Can you work these out from the model? Positions are in its coordinate system, mm. A direction names the side the tool comes from. Give positions to 0.01 mm unless a question says otherwise; leave off trailing zeros. Loops run counter-clockwise (first coordinate to the right, second up) from the corner with the lowest first, then second, coordinate; pieces in that order, holes last. Notation, with made-up numbers: (-39.75, 33.25) - (-33.75, 33.25) arc R23 ccw to (-33.75, 72.25) - close; hole circle Ø3 at (77, 37.25). An arc over 180 degrees is marked (long way). Answer as a JSON object with one key per item and string values.
```python
from build123d import *

# Parameters (mm, degrees)
SKETCH1_R                = 25
SKETCH1_R_2              = 16
BOSS_EXTRUDE1_DEPTH      = 45
BOSS_EXTRUDE2_DEPTH      = 10
BOSS_EXTRUDE3_DEPTH      = 35
FILLET1_R                = 12
FILLET2_R                = 12
FILLET3_R                = 6
FILLET4_R                = 12
FILLET5_R                = 3
FILLET6_R                = 6
BOSS_EXTRUDE4_DEPTH      = 48
BOSS_EXTRUDE4_DEPTH_BACK = 48
SKETCH2_R                = 19
SKETCH2_R_2              = 10
BOSS_EXTRUDE5_DEPTH      = 45
BOSS_EXTRUDE5_DEPTH_BACK = 45
SKETCH3_W                = 70
SKETCH3_H                = 86.046908332
CUT_EXTRUDE1_DEPTH       = 138.818721515
FILLET7_R                = 6
SKETCH4_R                = 5
CUT_EXTRUDE2_DEPTH       = 132.658649545
SKETCH6_R                = 19
SKETCH6_R_2              = 10
BOSS_EXTRUDE7_DEPTH      = 16
SKETCH7_R                = 19
SKETCH7_R_2              = 10
BOSS_EXTRUDE8_DEPTH      = 16


with BuildPart() as part:
    # Sketch1 → Boss-Extrude1 (new body)
    with BuildSketch(Plane(origin=(0, 0, 0), x_dir=(1, 0, 0), z_dir=(0, 1, 0))):
        with Locations(Location((0, 0, 0), (0, 0, 90))):
            Circle(SKETCH1_R)
        with Locations(Location((0, 0, 0), (0, 0, 90))):
            Circle(SKETCH1_R_2, mode=Mode.SUBTRACT)
    extrude(amount=BOSS_EXTRUDE1_DEPTH)

    # Sketch1<3> → Boss-Extrude2 (add)
    with BuildSketch(Plane(origin=(0, 0, 0), x_dir=(1, 0, 0), z_dir=(0, 1, 0))):
        with BuildLine():
            Line((-45, 50), (-69, 50))
            Line((-69, 50), (-69, 12))
            Line((-69, 12), (-45, 12))
            Line((-45, 12), (-45, -28))
            Line((-45, -28), (45, -28))
            Line((45, -28), (45, 12))
            Line((45, 12), (69, 12))
            Line((69, 12), (69, 50))
            Line((69, 50), (45, 50))
            Line((45, 50), (45, 25))
            Line((45, 25), (25, 25))
            Line((25, 25), (25, 0))
            ThreePointArc((25, 0), (0, -25), (-25, 0))
            Line((-25, 0), (-25, 25))
            Line((-25, 25), (-45, 25))
            Line((-45, 25), (-45, 50))
        make_face()
    extrude(amount=BOSS_EXTRUDE2_DEPTH)

    # Sketch1<4> → Boss-Extrude3 (add)
    with BuildSketch(Plane(origin=(0, 0, 0), x_dir=(1, 0, 0), z_dir=(0, 1, 0))):
        with BuildLine():
            Line((-35, 35), (-35, 60))
            Line((-35, 60), (-75, 60))
            Line((-75, 60), (-75, 50))
            Line((-75, 50), (-69, 50))
            Line((-69, 50), (-45, 50))
            Line((-45, 50), (-45, 25))
            Line((-45, 25), (-25, 25))
            Line((-25, 25), (-25, 0))
            ThreePointArc((-25, 0), (0, 25), (25, 0))
            Line((25, 0), (25, 25))
            Line((25, 25), (45, 25))
            Line((45, 25), (45, 50))
            Line((45, 50), (69, 50))
            Line((69, 50), (75, 50))
            Line((75, 50), (75, 60))
            Line((75, 60), (35, 60))
            Line((35, 60), (35, 35))
            Line((35, 35), (-35, 35))
        make_face()
    extrude(amount=BOSS_EXTRUDE3_DEPTH)

    # Fillet1
    fillet1_edges = [part.edges().sort_by_distance(p)[0] for p in [
        (45, 22.5, -25),
        (-45, 22.5, -25),
    ]]
    fillet(fillet1_edges, radius=FILLET1_R)

    # Fillet2
    fillet2_edges = [part.edges().sort_by_distance(p)[0] for p in [
        (-45, 5, -12),
        (45, 5, -12),
    ]]
    fillet(fillet2_edges, radius=FILLET2_R)

    # Fillet3
    fillet3_edges = [part.edges().sort_by_distance(p)[0] for p in [
        (69, 5, -50),
        (-69, 5, -50),
    ]]
    fillet(fillet3_edges, radius=FILLET3_R - 0.0001)  # a hair under: the kernel refuses the full size

    # Fillet4
    fillet4_edges = [part.edges().sort_by_distance(p)[0] for p in [
        (69, 5, -12),
        (-69, 5, -12),
    ]]
    fillet(fillet4_edges, radius=FILLET4_R - 0.0001)  # a hair under: the kernel refuses the full size

    # Fillet5
    fillet5_edges = [part.edges().sort_by_distance(p)[0] for p in [
        (25, 22.5, -25),
        (35, 17.5, -35),
        (-35, 17.5, -35),
        (-25, 22.5, -25),
    ]]
    fillet(fillet5_edges, radius=FILLET5_R)

    # Fillet6
    fillet6_edges = [part.edges().sort_by_distance(p)[0] for p in [
        (45, 22.5, -50),
        (-45, 22.5, -50),
    ]]
    fillet(fillet6_edges, radius=FILLET6_R)



with BuildPart() as body_2:
    # Sketch2 → Boss-Extrude4 (new, two sides: drawn at the far end of the back side and taken through both)
    with BuildSketch(Plane(origin=(0, 0, 0), x_dir=(0, 0, -1), z_dir=(1, 0, 0)).offset(-BOSS_EXTRUDE4_DEPTH_BACK)):
        with Locations((0, -56)):
            Circle(SKETCH2_R)
        with Locations((0, -56)):
            Circle(SKETCH2_R_2, mode=Mode.SUBTRACT)
    extrude(amount=BOSS_EXTRUDE4_DEPTH + BOSS_EXTRUDE4_DEPTH_BACK)


with BuildPart() as part_1:
    add(part.part)

    add(body_2.part)  # Boss-Extrude5 merges body 2
    # Sketch2<4> → Boss-Extrude5 (add, two sides: drawn at the far end of the back side and taken through both)
    with BuildSketch(Plane(origin=(0, 0, 0), x_dir=(0, 0, -1), z_dir=(1, 0, 0)).offset(-BOSS_EXTRUDE5_DEPTH_BACK)):
        with BuildLine():
            Line((0, 0), (-28, 0))
            Line((-28, 0), (-18.771282059, -58.939212458))
            ThreePointArc((-18.771282059, -58.939212458), (-1.474048996, -37.057265785), (19, -56))
            ThreePointArc((19, -56), (18.868026287, -58.235527685), (18.473938523, -60.439999487))
            Line((18.473938523, -60.439999487), (33, 0))
            Line((33, 0), (24, 0))
            Line((24, 0), (12, 0))
            Line((12, 0), (0, 0))
        make_face()
    extrude(amount=BOSS_EXTRUDE5_DEPTH + BOSS_EXTRUDE5_DEPTH_BACK)

    # Sketch3 → Cut-Extrude1 (cut, through all)
    with BuildSketch(Plane.XY.offset(28)):
        with Locations((0, -43.023454166)):
            Rectangle(SKETCH3_W, SKETCH3_H)
    extrude(amount=-CUT_EXTRUDE1_DEPTH, mode=Mode.SUBTRACT)

    # Fillet7
    fillet7_edges = [part_1.edges().sort_by_distance(p)[0] for p in [
        (-35, 0, -2.5),
        (35, 0, -2.5),
    ]]
    fillet(fillet7_edges, radius=FILLET7_R)

    # Sketch4 → Cut-Extrude2 (cut, through all)
    with BuildSketch(Plane.XY.offset(-50)):
        with Locations((-63, 23)):
            Circle(SKETCH4_R)
        with Locations((62.999455964, 23)):
            Circle(SKETCH4_R)
    extrude(amount=-CUT_EXTRUDE2_DEPTH, mode=Mode.SUBTRACT)

    # Sketch6 → Boss-Extrude7 (add)
    with BuildSketch(Plane(origin=(-32, 0, 0), x_dir=(0, 0, -1), z_dir=(1, 0, 0))):
        with Locations((0, -56)):
            Circle(SKETCH6_R)
        with Locations((0, -56)):
            Circle(SKETCH6_R_2, mode=Mode.SUBTRACT)
    extrude(amount=-BOSS_EXTRUDE7_DEPTH)

    # Sketch7 → Boss-Extrude8 (add)
    with BuildSketch(Plane.ZY.offset(-32)):
        with Locations(Location((0, -56, 0), (0, 0, 180))):
            Circle(SKETCH7_R)
        with Locations(Location((0, -56, 0), (0, 0, 180))):
            Circle(SKETCH7_R_2, mode=Mode.SUBTRACT)
    extrude(amount=-BOSS_EXTRUDE8_DEPTH)


solid = part_1.part
```
1) Which directions (+Z, -Z, +X, -X, +Y, -Y) give clear straight access to the entire face, cutting with the end or side of a thin tool? Please do faces 1 (the flat face through (0, 17, -35)), 2 (the flat face through (30, 22, -25)), 3 (the flat face through (-45, 22, -41)).
Check sheet entries:
{"face 1": "-Z, +Y, -Y", "face 2": "+Z, +X, +Y", "face 3": "+Z, -X, +Y"}
2) If we mould it in two halves opening along Y, with no side actions, what happens to faces 4 (the cylindrical face through (70.711, 5.07, -48.196)), 5 (the flat face through (16.3, 45, 0.4)), 6 (the cylindrical face through (61.916, 18.119, -54.93))? For each: released by +Y, released by -Y, zero draft, split by the parting line, or undercut.
Check sheet entries:
{"face 4": "zero draft", "face 5": "released by +Y", "face 6": "undercut"}
3) Imagine slicing it at D-D on x = -20. Write out the boundary of the cut face in (y, z), and give its area (3 significant figures).
Check sheet entries:
{"outline": "(0, -35) - (35, -35) - (35, -15) - (45, -15) - (45, 15) - (10, 15) - (10, 28) - (0, 28) - close", "area": "2,180 mm2"}
4) I need wall thicknesses on L1, parallel to X at y = -55, z = -14.5; L2, parallel to Y at x = 42, z = 0; L3, parallel to X at y = 20.5, z = 0. Which ranges of each line are inside material? Lowest first, please.
Check sheet entries:
{"L1": "-48 to -32, 32 to 48", "L2": "-75 to -66, -46 to 10", "L3": "-25 to -16, 16 to 25"}
5) I'm going to push flat-ended pins straight in: P1, Ø12, axis at x = -2, z = -16.5, coming from the -Y side; P2, Ø12, axis at y = -10, z = 4, coming from the +X side; P3, Ø18.5, axis at y = -16.5, z = 0.5, coming from the -X side; P4, Ø8, axis at y = -52, z = 1.5, coming from the -X side. Where does each tip first touch, or does it pass through?
Check sheet entries:
{"P1": "y = 0", "P2": "x = 45", "P3": "x = -45", "P4": "through"}
6) Imagine slicing it at A-A on y = 23. Give the number of separate pieces and of enclosed holes in the cut face, and give its area (3 significant figures).
Check sheet entries:
{"separate pieces": "3", "enclosed holes": "1", "area": "3,190 mm2"}
7) Imagine slicing it at B-B on x = 0. Write out the boundary of the cut face in (y, z).
Check sheet entries:
{"outline": "(0, -35) - (35, -35) - (35, -25) - (45, -25) - (45, -16) - (0, -16) - close; (0, 16) - (45, 16) - (45, 25) - (10, 25) - (10, 28) - (0, 28) - close"}
